Verification items for the finished model (mm, model axes). A direction names the side the tool comes from. Coordinates: 2 decimals unless noted, no trailing zeros. Loops run counter-clockwise (first coordinate to the right, second up) from the corner with the lowest first, then second, coordinate; pieces in that order, holes last. Notation, with made-up numbers: (55.5, -11) -> (89.5, -11) arc R33 cw to (89.5, 27) -> close; hole circle Ø9 at (-26.5, -36.5). An arc over 180 degrees is marked (long way). Write item = value, one per line.
Autodesk Inventor part; units mm, degrees
ref_plane "Work Plane1" through (0, 0, 0) normal (0, 1, 0) x (-1, 0, 0)
ref_plane "Work Plane2" through (0, 20, 0) normal (0, 1, 0) x (-1, 0, 0)
ref_plane "YZ Plane" through (0, 0, 0) normal (1, 0, 0) x (0, 1, 0)
sketch "Sketch2" plane through (0, 0, 0) normal (0, 1, 0) x (-1, 0, 0)
  arc A0 (-18.7617, -18) -> (-18.7617, 18) centre (0, 0) ccw
  arc A1 (-14.8324, -6) -> (-14.8324, 6) centre (0, 0) ccw
  line L0 (-16, 0) -> (-16, -6)
  line L1 (-16, 0) -> (-16, 6)
  line L2 (-16, 6) -> (-14.8324, 6) construction
  line L3 (-16, -6) -> (-14.8324, -6)
  circle A2 centre (22, 0) radius 1.5
  circle A3 centre (15.5563, 15.5563) radius 1.5
  circle A4 centre (0, 22) radius 1.5
  circle A5 centre (-15.5563, 15.5563) radius 1.5
  circle A6 centre (-22, 0) radius 1.5
  circle A7 centre (-15.5563, -15.5563) radius 1.5
  circle A8 centre (0, -22) radius 1.5
  circle A9 centre (15.5563, -15.5563) radius 1.5
  line L4 (-14.8324, 6) -> (-16, 6)
  line L5 (-30, 0) -> (-30, -18)
  line L6 (-30, -18) -> (-30, 18)
  line L7 (-30, 18) -> (-18.7617, 18)
  line L8 (-30, -18) -> (-18.7617, -18)
  arc A10 (-21.9489, 1.4991) -> (-22, 0) centre (0, 0) ccw
  line L9 (0, 0) -> (-16, 0)
  line L10 (-20.5, 0) -> (-22, 0)
  dimension "d10" = 360
  dimension "d2" = 52
  dimension "d3" = 32
  dimension "d4" = 6
  dimension "d5" = 6
  dimension "d6" = 3
  dimension "d7" = 30
  dimension "d8" = 18
  dimension "d9" = 36
  dimension "d36" = 22
  dimension "d37" = 0
  dimension "d38" = 18
  dimension "d39" = 0
  dimension "d40" = 16
  dimension "d41" = 38
extrude "Extrusion1" add sketch "Sketch2" along normal blind 40
ref_plane "Work Plane1" through (0, 0, 0) normal (0, 1, 0) x (-1, 0, 0)
sketch "Sketch6" plane through (0, 0, 0) normal (0, 1, 0) x (-1, 0, 0)
  arc A0 (-6.0828, -18) -> (-6.0828, 18) centre (0, 0) ccw
  circle A1 centre (0, 0) radius 26
  arc A2 (-18.7617, -18) -> (-18.7617, 18) centre (0, 0) ccw
  line L0 (-18.7617, 18) -> (-6.0828, 18)
  line L1 (-18.7617, -18) -> (-6.0828, -18)
  dimension "d31" = 38
  dimension "d32" = 52
  dimension "d73" = 26
  dimension "d74" = 36
  dimension "d75" = 18
  dimension "d76" = 18
  dimension "d77" = 0
sketch "Sketch4" plane through (30, 0, 18) normal (1, 0, 0) x (0, 0, -1)
  circle A0 centre (12, 3) radius 1.5
  circle A1 centre (3.5, 12) radius 1.5
  line L0 (0, 3) -> (0, 37) construction
  line L1 (0, 20) -> (36, 20) construction
  circle A2 centre (3.5, 28) radius 1.5
  circle A3 centre (12, 37) radius 1.5
  line L2 (16.5, 40) -> (19.5, 40) construction
  line L3 (18, 40) -> (18, 0) construction
  line L4 (19.5, 0) -> (16.5, 0) construction
  circle A4 centre (24, 37) radius 1.5
  circle A5 centre (32.5, 28) radius 1.5
  circle A6 centre (32.5, 12) radius 1.5
  circle A7 centre (24, 3) radius 1.5
  line L5 (-1, 37) -> (-1, 3)
  line L6 (37, 37) -> (37, 3)
  arc A8 (11.25, 21.5) -> (11.25, 18.5) centre (11.25, 20) ccw
  arc A9 (24.75, 18.5) -> (24.75, 21.5) centre (24.75, 20) ccw
  line L7 (24.75, 21.5) -> (24.75, 23)
  arc A10 (24.75, 23) -> (24.75, 25.5) centre (24.75, 24.25) ccw
  arc A11 (11.25, 25.5) -> (11.25, 23) centre (11.25, 24.25) ccw
  line L8 (24.75, 14.5) -> (11.25, 14.5)
  line L9 (24.75, 17) -> (11.25, 17)
  arc A12 (11.25, 17) -> (11.25, 14.5) centre (11.25, 15.75) ccw
  arc A13 (24.75, 14.5) -> (24.75, 17) centre (24.75, 15.75) ccw
  line L10 (11.25, 21.5) -> (24.75, 21.5)
  line L11 (24.75, 18.5) -> (11.25, 18.5)
  line L12 (11.25, 25.5) -> (24.75, 25.5)
  line L13 (11.25, 23) -> (24.75, 23)
  point P0 (18, 0)
  point P1 (0, 40)
  point P2 (36, 3)
  point P3 (18, 0)
  dimension "d18" = 3
  dimension "d21" = 3
  dimension "d22" = 3
  dimension "d23" = 1.5
  dimension "d24" = 2.5
  dimension "d25" = 2.5
  dimension "d26" = 2.5
  dimension "d42" = 12.25
  dimension "d43" = 19
  dimension "d44" = 37
  dimension "d45" = 38
  dimension "d46" = 25.5
  dimension "d47" = 20
  dimension "d48" = 17
  dimension "d49" = 40
  dimension "d50" = 19
  dimension "d51" = 0
  dimension "d52" = 37
  dimension "d53" = 3
  dimension "d54" = 1
  dimension "d55" = 1
  dimension "d56" = 3
  dimension "d57" = 4.5
  dimension "d58" = 28
  dimension "d59" = 12.25
  dimension "d60" = 13
  dimension "d61" = 37
  dimension "d62" = 17.5
  dimension "d63" = 17.5
  dimension "d64" = 19
  dimension "d65" = 0
  dimension "d66" = 25.75
  dimension "d67" = 25.75
  dimension "d68" = 37
  dimension "d69" = 40
  dimension "d70" = 37
  dimension "d71" = 37
  dimension "d72" = 3
extrude "Extrusion5" cut sketch "Sketch4" against normal blind 11
extrude "Extrusion6" cut sketch "Sketch6" along normal blind 34 contours A0 L0 A1 L1 picked at (-12.9468, 19.3038)
ref_plane "Work Plane2" through (0, 20, 0) normal (0, 1, 0) x (-1, 0, 0)
mirror "Mirror1" about plane through (0, 20, 0) normal (0, 1, 0)
sketch "Sketch9" plane through (18.7617, 40, 18) normal (0, 0, 1) x (1, 0, 0)
  line L0 (-12.6789, -34) -> (0, -34)
  line L1 (0, -34) -> (0, -40)
  line L2 (11.2383, -40) -> (0, -40)
  line L3 (11.2383, -40) -> (11.2383, 0)
  line L4 (0, 0) -> (11.2383, 0)
  line L5 (0, -6) -> (0, 0)
  line L6 (0, -6) -> (-12.6789, -6)
  line L7 (-12.6789, -34) -> (-12.6789, -6)
  line L8 (11.2383, -18.5) -> (0.2383, -18.5)
  circle A0 centre (0.2383, -18.5) radius 2.25
  point P0 (-18.7617, -40)
  dimension "d81" = 4.5
extrude "Extrusion8" cut sketch "Sketch9" against normal blind 10 contours A0
properties part number "reverse gear cylinder"
1) Sectioned sample at A-A, the plane x = 0. Count the separate pieces of the cut face and the enclosed holes in it, plus the area to 3 significant figures.
Ans:
separate_pieces = 6
enclosed_holes = 0
area = 336 mm2
2) Tool access check on faces 4 (the face through (19, 20, 0)), 5 (the face through (18, 20, -18)), 6 (the face through (21.08, 20.64, 13.07)), 7 (the face through (-25.986, 36.958, 0.865)). Record the directions out of +Z, -Z, +X, -X, +Y, -Y that give a thin tool (end or side, any length) a straight path to the whole face; none if there is none.
Ans:
face_4 = +X
face_5 = -Z, +X
face_6 = +Z
face_7 = +Y, -Y
3) Material ranges on line 1 (Z direction, x = 0, y = 2); line 2 (X direction, y = 22.45, z = 0); line 3 (X direction, y = 3.55, z = 0), recorded low to high.
Ans:
line_1 = -26 to -23.5, -20.5 to -16, 16 to 20.5, 23.5 to 26
line_2 = -19 to -16, 16 to 20.5, 23.5 to 30
line_3 = -26 to -23.5, -20.5 to -16, 16 to 20.5, 23.5 to 30
4) Sectioned sample at B-B, the plane z = 22. Record the cut outline in (x, y).
Ans:
outline = (-13.86, 0) -> (-1.5, 0) -> (-1.5, 6) -> (-13.86, 6) -> close; (-13.86, 34) -> (-1.5, 34) -> (-1.5, 40) -> (-13.86, 40) -> close; (1.5, 0) -> (13.86, 0) -> (13.86, 6) -> (1.5, 6) -> close; (1.5, 34) -> (13.86, 34) -> (13.86, 40) -> (1.5, 40) -> close
5) Depth check by flat-ended pin: pin 1 Ø1.8 at (y, z) = (37, -6) entering from +X; pin 2 Ø4 at (x, y) = (-4, 4.5) entering from -Z; pin 3 Ø0.6 at (x, y) = (15.5, 14) entering from +Z. Enter the tip coordinate at first touch or a pass-through.
Ans:
pin_1 = 19
pin_2 = -25.92
pin_3 = 18
6) Release check for a two-part mould opening along Y. For faces 1 (the face through (-20.5, 3.04, 0.07)), 2 (the face through (15, 40, 12)), 3 (the face through (19, 3, 6)) record: pulls with the +Y half, pulls with the -Y half, needs draft (parallel to the pull), parting line crosses it, or undercut.
Ans:
face_1 = needs draft
face_2 = pulls with the +Y half
face_3 = undercut
7) Sectioned sample at D-D, the plane y = 32.5. Record the cut outline in (x, z), plus the area to 3 significant figures.
Ans:
outline = (6.08, -18) -> (30, -18) -> (30, 18) -> (6.08, 18) arc R19 ccw (long way) to start; hole circle Ø3 at (15.56, -15.56); hole circle Ø3 at (15.56, 15.56); hole (14.83, -6) -> (16, -6) -> (16, 6) -> (14.83, 6) arc R16 ccw (long way) to start; hole circle Ø3 at (22, 0)
area = 825 mm2
8) Sectioned sample at C-C, the plane z = -10. Record the cut outline in (x, y).
Ans:
outline = (-24, 0) -> (-12.49, 0) -> (-12.49, 40) -> (-24, 40) -> (-24, 34) -> (-16.16, 34) -> (-16.16, 6) -> (-24, 6) -> close; (12.49, 0) -> (30, 0) -> (30, 40) -> (12.49, 40) -> close
